```python
from build123d import *

# Parameters (mm, degrees)
ESQUISSE1_R             = 1.5
ESQUISSE1_R_2           = 34.4618877
BOSS_EXTRU_1_DEPTH      = 5
ENL_V_MAT_EXTRU_1_REACH = 178.814
ESQUISSE2_W             = 10
ESQUISSE2_H             = 15


with BuildPart() as part:
    # Esquisse1 → Boss.-Extru.1 (new body)
    with BuildSketch(Plane(origin=(0, 0, 0), x_dir=(1, 0, 0), z_dir=(0, 1, 0))):
        with BuildLine():
            Line((-97.415, -97.504460786), (0, -97.504460786))
            Line((0, -97.504460786), (0, -40.004460786))
            ThreePointArc((0, -40.004460786), (-40, -0.004460786), (0, 39.995539214))
            Line((0, 39.995539214), (0, 97.495539214))
            Line((0, 97.495539214), (-97.415, 97.495539214))
            Line((-97.415, 97.495539214), (-97.415, 47.495539214))
            Line((-97.415, 47.495539214), (-147.415, 47.495539214))
            Line((-147.415, 47.495539214), (-147.415, -47.504460786))
            Line((-147.415, -47.504460786), (-97.415, -47.504460786))
            Line((-97.415, -47.504460786), (-97.415, -97.504460786))
        make_face()
        with Locations(Location((-142.415, -12.504460786, 0), (0, 0, 270))):
            Circle(ESQUISSE1_R, mode=Mode.SUBTRACT)
        with Locations(Location((-92.415, -42.504460786, 0), (0, 0, 270))):
            Circle(ESQUISSE1_R, mode=Mode.SUBTRACT)
        with Locations(Location((-12.415, -92.504460786, 0), (0, 0, 270))):
            Circle(ESQUISSE1_R, mode=Mode.SUBTRACT)
        with Locations(Location((-31.819805153, -29.234805153, 0), (0, 0, 270))):
            Circle(ESQUISSE1_R, mode=Mode.SUBTRACT)
        with Locations(Location((-142.415, 12.495539214, 0), (0, 0, 270))):
            Circle(ESQUISSE1_R, mode=Mode.SUBTRACT)
        with Locations(Location((-100.973221988, -0.004460786, 0), (0, 0, 270))):
            Circle(ESQUISSE1_R_2, mode=Mode.SUBTRACT)
        with Locations(Location((-92.415, 42.495539214, 0), (0, 0, 270))):
            Circle(ESQUISSE1_R, mode=Mode.SUBTRACT)
        with Locations(Location((-31.819805153, 29.225883581, 0), (0, 0, 270))):
            Circle(ESQUISSE1_R, mode=Mode.SUBTRACT)
        with Locations(Location((-12.415, 92.495539214, 0), (0, 0, 270))):
            Circle(ESQUISSE1_R, mode=Mode.SUBTRACT)
    extrude(amount=BOSS_EXTRU_1_DEPTH)

    # Esquisse2 → Enlèv. mat.-Extru.1 (cut, up to next)
    with BuildSketch(Plane(origin=(0, 5, 0), x_dir=(1, 0, 0), z_dir=(0, 1, 0)), mode=Mode.PRIVATE) as enl_v_mat_extru_1_sk1:
        with Locations((-76.715147883, 77.495539214)):
            Rectangle(ESQUISSE2_W, ESQUISSE2_H)
    enl_v_mat_extru_1_tool1 = extrude(enl_v_mat_extru_1_sk1.sketch, amount=-ENL_V_MAT_EXTRU_1_REACH, mode=Mode.PRIVATE) & part.part
    # Esquisse2 → Enlèv. mat.-Extru.1 (cut, up to next)
    with BuildSketch(Plane(origin=(0, 5, 0), x_dir=(1, 0, 0), z_dir=(0, 1, 0)), mode=Mode.PRIVATE) as enl_v_mat_extru_1_sk2:
        with Locations((-46.715147883, 77.495539214)):
            Rectangle(ESQUISSE2_W, ESQUISSE2_H)
    enl_v_mat_extru_1_tool2 = extrude(enl_v_mat_extru_1_sk2.sketch, amount=-ENL_V_MAT_EXTRU_1_REACH, mode=Mode.PRIVATE) & part.part
    # Esquisse2 → Enlèv. mat.-Extru.1 (cut, up to next)
    with BuildSketch(Plane(origin=(0, 5, 0), x_dir=(1, 0, 0), z_dir=(0, 1, 0)), mode=Mode.PRIVATE) as enl_v_mat_extru_1_sk3:
        with Locations((-16.715147883, 77.495539214)):
            Rectangle(ESQUISSE2_W, ESQUISSE2_H)
    enl_v_mat_extru_1_tool3 = extrude(enl_v_mat_extru_1_sk3.sketch, amount=-ENL_V_MAT_EXTRU_1_REACH, mode=Mode.PRIVATE) & part.part
    add(enl_v_mat_extru_1_tool1.solids().sort_by_distance((-76.715148, 5, -77.495539))[0], mode=Mode.SUBTRACT)
    add(enl_v_mat_extru_1_tool2.solids().sort_by_distance((-46.715148, 5, -77.495539))[0], mode=Mode.SUBTRACT)
    add(enl_v_mat_extru_1_tool3.solids().sort_by_distance((-16.715148, 5, -77.495539))[0], mode=Mode.SUBTRACT)


solid = part.part
```
Geometry check sheet. Reference: the model listing, model coordinates, mm. A direction names the side the tool comes from. Coordinates: 2 decimals unless noted, no trailing zeros. Loops run counter-clockwise (first coordinate to the right, second up) from the corner with the lowest first, then second, coordinate; pieces in that order, holes last. Notation, with made-up numbers: (-30, -18.5) -> (-25, -18.5) arc R6 ccw to (-25, -8.5) -> close; hole circle Ø8 at (33, 28.25). An arc over 180 degrees is marked (long way). Put each result on its own line as item: value.
1) Release check for a two-part mould opening along X. For faces 5 (the flat face through (-58, 5, -1)), 6 (the flat face through (-147.415, 2, -1)), 7 (the flat face through (-51.715, 3, -77)), 8 (the cylindrical face through (-39.99, 2.46, 0.88)) record: released by +X, released by -X, zero draft, split by the parting line, or undercut.
Result set:
face 5: zero draft
face 6: released by -X
face 7: undercut
face 8: released by +X
2) Cross-section at A-A on z = 0. Record the boundary of the cut face in (x, y) (3 decimals), plus the area to 3 significant figures.
Result set:
outline: (-147.415, 0) -> (-135.435, 0) -> (-135.435, 5) -> (-147.415, 5) -> close; (-66.511, 0) -> (-40, 0) -> (-40, 5) -> (-66.511, 5) -> close
area: 192 mm^2
3) Thickness scan on line 1 (X direction, y = 4.5, z = -77.5) (3 decimals); line 2 (Z direction, x = -17, y = 2.4); line 3 (Z direction, x = -101.5, y = 4.65). Record the ranges inside material, lowest first.
Result set:
line 1: x = -97.415 to -81.715, -71.715 to -51.715, -41.715 to -21.715, -11.715 to 0
line 2: z = -97.5 to -85, -70 to -36.2, 36.21 to 97.5
line 3: z = -47.5 to -34.45, 34.46 to 47.5
4) Gauge pin test, flat ends, axial feed: pin 1 Ø3.5 at (x, z) = (-142.42, -12.5) entering from +Y; pin 2 Ø1 at (y, z) = (3, -50.5) entering from -X (3 decimals); pin 3 Ø1 at (x, y) = (-130.5, 1) entering from -Z. Record the tip position at first contact, or that the pin passes through.
Result set:
pin 1: stops at y = 5
pin 2: stops at x = -97.415
pin 3: stops at z = -47.5
5) Tool access check on faces 1 (the flat face through (0, 2, -68)), 2 (the flat face through (-97.415, 2, -73)), 3 (the flat face through (-123, 2, 47.504)), 4 (the flat face through (-47, 3, -69.996)). Record the directions out of +Z, -Z, +X, -X, +Y, -Y that give a thin tool (end or side, any length) a straight path to the whole face; none if there is none.
Result set:
face 1: +Z, -Z, +X, +Y, -Y
face 2: -Z, -X, +Y, -Y
face 3: +Z, -X, +Y, -Y
face 4: +Y, -Y
6) Cross-section at B-B on x = -77.5. Record the boundary of the cut face in (y, z).
Result set:
outline: (0, -97.5) -> (5, -97.5) -> (5, -85) -> (0, -85) -> close; (0, -70) -> (5, -70) -> (5, -25.23) -> (0, -25.23) -> close; (0, 25.24) -> (5, 25.24) -> (5, 97.5) -> (0, 97.5) -> close
7) Cross-section at C-C on y = 1.6. Count the separate pieces of the cut face and the enclosed holes in it, plus the area to 3 significant figures.
Result set:
separate pieces: 1
enclosed holes: 12
area: 17,000 mm^2
8) Cross-section at D-D on x = -125.5. Record the boundary of the cut face in (y, z), plus the area to 3 significant figures.
Result set:
outline: (0, -47.5) -> (5, -47.5) -> (5, -24.2) -> (0, -24.2) -> close; (0, 24.21) -> (5, 24.21) -> (5, 47.5) -> (0, 47.5) -> close
area: 233 mm^2
